Check sheet for the modelled part. Datum: model origin and axes. Units: mm. A direction names the side the tool comes from. Round coordinates to 2 decimals unless told otherwise and drop trailing zeros. Write each loop counter-clockwise with the first axis right and the second up, starting at its lowest first coordinate (ties: lowest second). Pieces come first, ordered by that corner, then holes.
Item 1: Material ranges on line 1 (X direction, y = -177, z = 41); line 2 (Y direction, x = 177, z = 41); line 3 (X direction, y = 105.5, z = 2), recorded low to high.
Item 2: Go/stop test with flat-tipped pins: pin 1 Ø6.5 at (x, z) = (-119.29, 41) entering from -Y; pin 2 Ø1.4 at (y, z) = (-177, 28) entering from +X; pin 3 Ø2.5 at (x, z) = (177, 29) entering from -Y; pin 4 Ø6 at (x, z) = (-160, 41) entering from +Y. Record where each tip stops, or that it passes through.
Item 3: Cross-section at C-C on y = -106. Enter the section's corners in (x, z), plus the area to 3 significant figures.
Item 4: Tool access check on faces 1 (the flat face through (175.737, 139, 29)), 2 (the flat face through (-140, -179.737, 28)), 3 (the flat face through (-140, -175.737, 29)). Record the directions out of +Z, -Z, +X, -X, +Y, -Y that give a thin tool (end or side, any length) a straight path to the whole face; none if there is none.
Item 5: Cross-section at A-A on z = 13. Enter the section's corners in (x, y), plus the area to 3 significant figures.
Item 6: Cross-section at B-B on x = 89.5. Enter the section's corners in (y, z).
from build123d import *

# Parameters (mm, degrees)
BASE_FLANGE1_DEPTH      = 4
EDGE_FLANGE1_DEPTH      = 70.710678119
EDGE_FLANGE1_BEND_DEPTH = 70.710678119
SKETCH13_R              = 2.55
CUT_EXTRUDE1_DEPTH      = 4
SKETCH14_R              = 2.55
CUT_EXTRUDE2_DEPTH      = 4
FILLET1_R               = 5


# Sheet-metal steps are written as plain solids
with BuildPart() as part:
    # Sketch1 → Base-Flange1 (new body)
    with BuildSketch(Plane.XY):
        Polygon((175, 175), (-175, -175), (-104.289321881, -175), (175, 104.289321881), align=None)
    extrude(amount=-BASE_FLANGE1_DEPTH)

    # Edge-Flange1 section (across the edge) → Edge-Flange1 (add)
    with BuildSketch(Plane(origin=(175.7366, 104.289321881, 0), x_dir=(-1, 0, 0), z_dir=(0, 1, 0))):
        with BuildLine():
            Line((-4, 0.7366), (-4, 56))
            Line((-4, 56), (0, 56))
            Line((0, 56), (0, 0.7366))
            ThreePointArc((0, 0.7366), (0.215745145, 0.215745145), (0.7366, 0))
            Line((0.7366, 0), (0.7366, -4))
            ThreePointArc((0.7366, -4), (-2.61268198, -2.61268198), (-4, 0.7366))
        make_face()
    extrude(amount=EDGE_FLANGE1_DEPTH)

    # Edge-Flange1 section 2 (across the edge) → Edge-Flange1 bend (add)
    with BuildSketch(Plane(origin=(-175, -175.7366, 0), x_dir=(0, 1, 0), z_dir=(1, 0, 0))):
        with BuildLine():
            Line((-4, 0.7366), (-4, 56))
            Line((-4, 56), (0, 56))
            Line((0, 56), (0, 0.7366))
            ThreePointArc((0, 0.7366), (0.215745145, 0.215745145), (0.7366, 0))
            Line((0.7366, 0), (0.7366, -4))
            ThreePointArc((0.7366, -4), (-2.61268198, -2.61268198), (-4, 0.7366))
        make_face()
    extrude(amount=EDGE_FLANGE1_BEND_DEPTH)

    # Sketch13 → Cut-Extrude1 (cut)
    with BuildSketch(Plane(origin=(179.7366, 0, 0), x_dir=(0, 0, -1), z_dir=(1, 0, 0))):
        with Locations((-41, 160)):
            Circle(SKETCH13_R)
        with Locations(Location((-41, 119.289321881, 0), (0, 0, 180))):
            Circle(SKETCH13_R)
    extrude(amount=-CUT_EXTRUDE1_DEPTH, mode=Mode.SUBTRACT)

    # Sketch14 → Cut-Extrude2 (cut)
    with BuildSketch(Plane.XZ.offset(179.7366)):
        with Locations(Location((-119.289321881, 41, 0), (0, 0, 270))):
            Circle(SKETCH14_R)
        with Locations(Location((-160, 41, 0), (0, 0, 90))):
            Circle(SKETCH14_R)
    extrude(amount=-CUT_EXTRUDE2_DEPTH, mode=Mode.SUBTRACT)

    # Fillet1
    fillet1_edges = [part.edges().sort_by_distance(p)[0] for p in [
        (177.7366, 104.289321881, 56),
        (177.7366, 175, 56),
        (-175, -177.7366, 56),
        (-104.289321881, -177.7366, 56),
    ]]
    fillet(fillet1_edges, radius=FILLET1_R)


solid = part.part
Response values:
1. line 1: x = -175 to -162.55, -157.45 to -121.84, -116.74 to -104.29
1. line 2: y = 104.29 to 116.74, 121.84 to 157.45, 162.55 to 175
1. line 3: x = 175.74 to 179.74
2. pin 1: stops at y = -179.74
2. pin 2: stops at x = -104.29
2. pin 3: stops at y = 104.29
2. pin 4: stops at y = -175.74
3. outline: (-106, -4) - (-35.29, -4) - (-35.29, 0) - (-106, 0) - close
3. area: 283 mm2
4. face 1: +Z, -X, +Y, -Y
4. face 2: +Z, -Z, +X, -X, -Y
4. face 3: +Z, +X, -X, +Y
5. outline: (-175, -179.74) - (-104.29, -179.74) - (-104.29, -175.74) - (-175, -175.74) - close; (175.74, 104.29) - (179.74, 104.29) - (179.74, 175) - (175.74, 175) - close
5. area: 566 mm2
6. outline: (18.79, -4) - (89.5, -4) - (89.5, 0) - (18.79, 0) - close
